For this review, take the finished solid that the model builds, in its own axes (mm). Round coordinates to 2 decimals unless told otherwise and drop trailing zeros. Loops run counter-clockwise (first coordinate to the right, second up) from the corner with the lowest first, then second, coordinate; pieces in that order, holes last.
1) Take a section at A-A (x = 75). State the section outline as (y, z) points.
2) Insertion check: pin 1 (4 mm diameter, centred on x = -53.63, y = 18.14, fed in from -Z) (3 decimals). The pin has a flat end and moves straight along its axis. Give the tip position at first contact, or say it passes through.
3) Mouldability with a two-part tool opening along Y and no side actions: class faces 1 (the flat face through (10, 0, 3)), 2 (the flat face through (10, 36.27, 3)), 3 (the cylindrical face through (74.226, 19.825, 2.687)), 4 (the flat face through (-76.282, 18, 3)) as pulls with the +Y half, pulls with the -Y half, needs draft (parallel to the pull), parting line crosses it, or undercut.
4) Wall thickness on L1, parallel to X at y = 16, z = 2.5; L2, parallel to Y at x = 74, z = 1.3: over which ranges is each line inside the solid? List them lowest first.
```python
from build123d import *

# Parameters (mm, degrees)
ESQUISSE2_W             = 175
ESQUISSE2_H             = 3
BOSS_EXTRU_1_DEPTH      = 36.27
ESQUISSE3_R             = 2.5
ENL_V_MAT_EXTRU_1_DEPTH = 106.213182302


with BuildPart() as part:
    # Esquisse2 → Boss.-Extru.1 (new body)
    with BuildSketch(Plane(origin=(0, 0, 0), x_dir=(1, 0, 0), z_dir=(0, 1, 0))):
        with Locations((11.218290251, -2.666038947)):
            Rectangle(ESQUISSE2_W, ESQUISSE2_H)
    extrude(amount=BOSS_EXTRU_1_DEPTH)

    # Esquisse3 → Enlèv. mat.-Extru.1 (cut, through all)
    with BuildSketch(Plane.XY.offset(4.166038947)):
        with Locations((-53.631709749, 18.135)):
            Circle(ESQUISSE3_R)
        with Locations((76.068290251, 18.135)):
            Circle(ESQUISSE3_R)
    extrude(amount=-ENL_V_MAT_EXTRU_1_DEPTH, mode=Mode.SUBTRACT)


solid = part.part
```
Response:
1. outline: (0, 1.17) - (15.87, 1.17) - (15.87, 4.17) - (0, 4.17) - close; (20.4, 1.17) - (36.27, 1.17) - (36.27, 4.17) - (20.4, 4.17) - close
2. pin 1: passes through
3. face 1: pulls with the -Y half
3. face 2: pulls with the +Y half
3. face 3: undercut
3. face 4: needs draft
4. L1: x = -76.28 to -54.93, -52.33 to 74.77, 77.37 to 98.72
4. L2: y = 0 to 16.73, 19.54 to 36.27
